```python
from build123d import *

# Parameters (mm, degrees)
SKETCH1_R           = 7
BOSS_EXTRUDE1_DEPTH = 3
SKETCH1_3_R         = 4
BOSS_EXTRUDE2_DEPTH = 55
SKETCH2_R           = 0.95
CUT_EXTRUDE1_DEPTH  = 57.524331044
CHAMFER1_SIZE       = 1


with BuildPart() as part:
    # Sketch1 → Boss-Extrude1 (new body)
    with BuildSketch(Plane(origin=(0, 0, 0), x_dir=(1, 0, 0), z_dir=(0, 1, 0))):
        with Locations(Location((0, 0, 0), (0, 0, 270))):
            Circle(SKETCH1_R)
    extrude(amount=-BOSS_EXTRUDE1_DEPTH)

    # Sketch1_3 → Boss-Extrude2 (add)
    with BuildSketch(Plane(origin=(0, 0, 0), x_dir=(1, 0, 0), z_dir=(0, 1, 0))):
        with Locations(Location((0, 0, 0), (0, 0, 270))):
            Circle(SKETCH1_3_R)
    extrude(amount=BOSS_EXTRUDE2_DEPTH)

    # Sketch2 → Cut-Extrude1 (cut, through all)
    with BuildSketch(Plane(origin=(0, 0, -4), x_dir=(-1, 0, 0), z_dir=(0, 0, -1))):
        with Locations(Location((0, 53, 0), (0, 0, 89.999999943))):
            Circle(SKETCH2_R)
    extrude(amount=-CUT_EXTRUDE1_DEPTH, mode=Mode.SUBTRACT)

    # Chamfer1
    chamfer1_edges = [part.edges().sort_by_distance(p)[0] for p in [
        (0, -3, -7),
    ]]
    chamfer(chamfer1_edges, length=CHAMFER1_SIZE)


solid = part.part
```
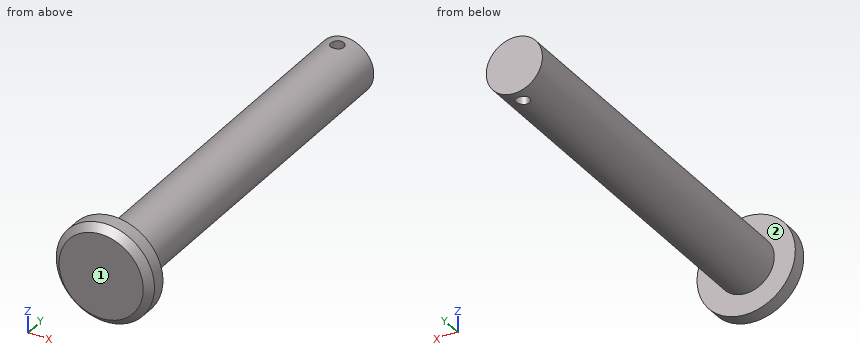
The model under review builds one solid part; all positions refer to its coordinate system, in mm. Face numbers are marked on the shaded views. A direction names the side the tool comes from. Give positions to 0.01 mm unless a question says otherwise; leave off trailing zeros. Write each loop counter-clockwise with the first axis right and the second up, starting at its lowest first coordinate (ties: lowest second). Pieces come first, ordered by that corner, then holes. Notation, with made-up numbers: (70, 15) -> (87, 15) arc R30 ccw to (87, 38) -> close; hole circle Ø4 at (71, -27). An arc over 180 degrees is marked (long way). Answer in a Markdown table with one row per item.
1) Add section C-C on y = 14. State the section outline as (x, z) points.
Worked answers:
| item | result |
|---|---|
| outline | circle Ø8 at (0, 0) |
2) Add section D-D on y = 53. State the section outline as (x, z) points, plus the area to 3 significant figures.
Worked answers:
| item | result |
|---|---|
| outline | (-0.95, -3.89) -> (-0.95, 3.89) arc R4 ccw to start; (0.95, -3.89) arc R4 ccw to (0.95, 3.89) -> close |
| area | 35.2 mm² |
3) For L1, parallel to Y at x = 0, z = 0.75; L2, parallel to Y at x = -4, z = -3.75; L3, parallel to X at y = 53, z = -0.25, list the stretches that pass through material, from the lowest coordinate up. Write a range as [from, to].
Worked answers:
| item | result |
|---|---|
| L1 | [-3, 52.05], [53.95, 55] |
| L2 | [-3, 0] |
| L3 | [-3.99, -0.95], [0.95, 3.99] |
4) Clearance check with flat-ended pins moving along their axes: P1, Ø2, axis at x = 2.5, y = 30, coming from the -Z side; P2, Ø2, axis at x = 0, y = 53, coming from the -Z side; P3, Ø7, axis at x = -3.5, z = -2.5, coming from the +Y side; P4, Ø6, axis at y = 10, z = -5, coming from the +X side. State where each tip first meets the part, or that it passes through.
Worked answers:
| item | result |
|---|---|
| P1 | z = -3.71 |
| P2 | z = -4 |
| P3 | y = 55 |
| P4 | x = 3.46 |
5) Add section A-A on x = 0. State the section outline as (y, z) points.
Worked answers:
| item | result |
|---|---|
| outline | (-3, -6) -> (-2, -7) -> (0, -7) -> (0, -4) -> (52.05, -4) -> (52.05, 4) -> (0, 4) -> (0, 7) -> (-2, 7) -> (-3, 6) -> close; (53.95, -4) -> (55, -4) -> (55, 4) -> (53.95, 4) -> close |
6) Add section B-B on z = 0. State the section outline as (x, y) points.
Worked answers:
| item | result |
|---|---|
| outline | (-7, -2) -> (-6, -3) -> (6, -3) -> (7, -2) -> (7, 0) -> (4, 0) -> (4, 55) -> (-4, 55) -> (-4, 0) -> (-7, 0) -> close; hole circle Ø1.9 at (0, 53) |
7) Tool access review of the marked faces 1 and 2: name each direction out of +Z, -Z, +X, -X, +Y, -Y from which nothing blocks a thin tool from reaching the whole face with its end or side.
Worked answers:
| item | result |
|---|---|
| face 1 | +Z, -Z, +X, -X, -Y |
| face 2 | +Y |
